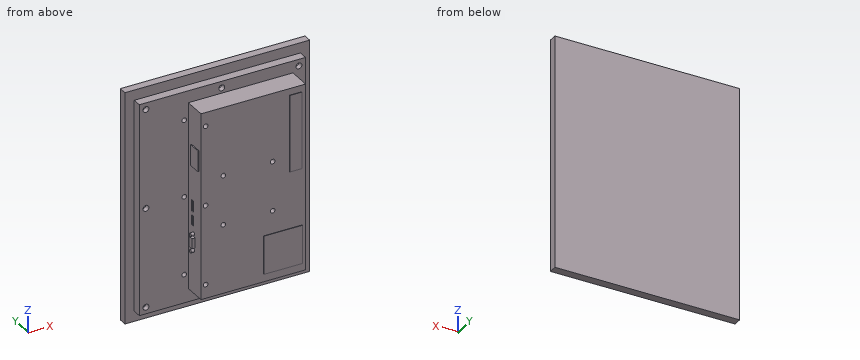
Autodesk Inventor part; units mm, degrees
ref_plane "YZ Plane" through (0, 0, 0) normal (1, 0, 0) x (0, 1, 0)
ref_plane "XZ Plane" through (0, 0, 0) normal (0, 1, 0) x (-1, 0, 0)
ref_plane "XY Plane" through (0, 0, 0) normal (0, 0, 1) x (1, 0, 0)
sketch "Sketch1" plane through (0, 0, 0) normal (0, 1, 0) x (-1, 0, 0)
  point P0 (0, 0)
sketch "Sketch2" plane through (0, 0, 0) normal (0, 1, 0) x (-1, 0, 0)
  line L0 (-139.5, 175.3) -> (139.5, 175.3)
  line L1 (139.5, 175.3) -> (139.5, -175.3)
  line L2 (139.5, -175.3) -> (-139.5, -175.3)
  line L3 (-139.5, -175.3) -> (-139.5, 175.3)
  line L4 (-139.5, 175.3) -> (139.5, -175.3) construction
  line L5 (139.5, 175.3) -> (-139.5, -175.3) construction
  point P0 (0, 0)
  dimension "d0" = 350.6
  dimension "d1" = 279
extrude "Extrusion1" add sketch "Sketch2" along normal blind 12.4
sketch "Sketch3" plane through (0, 0, 0) normal (0, -1, 0) x (1, 0, 0)
  line L0 (-125.5, -159.875) -> (125.5, -159.875)
  line L1 (125.5, -159.875) -> (125.5, 159.875)
  line L2 (125.5, 159.875) -> (-125.5, 159.875)
  line L3 (-125.5, 159.875) -> (-125.5, -159.875)
  line L4 (-125.5, -159.875) -> (125.5, 159.875) construction
  line L5 (125.5, -159.875) -> (-125.5, 159.875) construction
  point P0 (0, 0)
  dimension "d4" = 319.75
  dimension "d5" = 251
extrude "Extrusion2" add sketch "Sketch3" along normal blind 13.5
sketch "Sketch4" plane through (0, -13.5, 0) normal (0, -1, 0) x (1, 0, 0)
  line L0 (125.5, 159.875) -> (-125.5, 159.875)
  line L1 (-125.5, 159.875) -> (-125.5, -159.875)
  line L2 (125.5, -159.875) -> (125.5, 159.875)
  line L3 (-125.5, -159.875) -> (125.5, -159.875)
  point P0 (0, 0)
  point P1 (-115.5, 149.875)
  point P2 (-115.5, -149.875)
  point P3 (115.5, 149.875)
  point P4 (115.5, -149.875)
  dimension "d15" = 10
  dimension "d16" = 10
  dimension "d19" = 299.75
  dimension "d22" = 231
  dimension "d25" = 10
  dimension "d26" = 10
hole "Hole1" at (-115.5, -13.5, 149.875) at (115.5, -13.5, 149.875) at (115.5, -13.5, -149.875) at (-115.5, -13.5, -149.875) direction (0, 1, 0) diameter 9 depth 8 tip angle 118
sketch "Sketch5" plane through (0, -13.5, 0) normal (0, -1, 0) x (1, 0, 0)
  line L0 (125.5, 159.875) -> (-125.5, 159.875)
  line L1 (-125.5, 159.875) -> (-125.5, -159.875)
  line L2 (125.5, -159.875) -> (125.5, 159.875)
  point P0 (0, 0)
  point P1 (-115.5, 0)
  point P2 (115.5, 0)
  dimension "d34" = 159.875
  dimension "d35" = 10
  dimension "d38" = 231
  dimension "d43" = 10
hole "Hole2" at (-115.5, -13.5, 0) at (115.5, -13.5, 0) direction (0, 1, 0) diameter 9 depth 8 tip angle 118
sketch "Sketch6" plane through (0, -13.5, 0) normal (0, -1, 0) x (1, 0, 0)
  circle A0 centre (-115.5, 149.875) radius 4.5
  line L0 (-125.5, 159.875) -> (-125.5, -159.875)
  line L1 (-125.5, -159.875) -> (125.5, -159.875)
  line L2 (125.5, 159.875) -> (-125.5, 159.875)
  point P0 (0, 0)
  point P1 (-1, 149.875)
  point P2 (-1, -149.875)
  dimension "d55" = 298
  dimension "d52" = 124.5
  dimension "d60" = 10
  dimension "d188" = 10
hole "Hole3" at (-1, -13.5, -149.875) at (-1, -13.5, 149.875) direction (0, 1, 0) diameter 9 depth 8 tip angle 118
sketch "Sketch7" plane through (0, -13.5, 0) normal (0, -1, 0) x (1, 0, 0)
  line L0 (-51.5, 141.825) -> (106.5, 141.825)
  line L1 (106.5, 141.825) -> (106.5, -139.875)
  line L2 (106.5, -139.875) -> (-51.5, -139.875)
  line L3 (-51.5, -139.875) -> (-51.5, 141.825)
  line L4 (-51.5, 141.825) -> (106.5, -139.875) construction
  line L5 (106.5, 141.825) -> (-51.5, -139.875) construction
  line L6 (125.5, -159.875) -> (125.5, 159.875)
  line L7 (-125.5, -159.875) -> (125.5, -159.875)
  point P0 (0, 0)
  dimension "d61" = 281.7
  dimension "d62" = 158
  dimension "d63" = 19
  dimension "d64" = 20
extrude "Extrusion3" add sketch "Sketch7" along normal blind 33.6
sketch "Sketch8" plane through (0, -47.1, 0) normal (0, -1, 0) x (1, 0, 0)
  line L0 (100.2, 131.825) -> (82.2, 131.825)
  line L1 (82.2, 131.825) -> (82.2, 15.825)
  line L2 (82.2, 15.825) -> (100.2, 15.825)
  line L3 (100.2, 15.825) -> (100.2, 131.825)
  line L4 (100.2, 131.825) -> (82.2, 15.825) construction
  line L5 (82.2, 131.825) -> (100.2, 15.825) construction
  line L6 (106.5, -139.875) -> (106.5, 141.825)
  line L7 (106.5, 141.825) -> (-51.5, 141.825)
  point P0 (0, 0)
  point P1 (91.2, 73.825)
  dimension "d67" = 116
  dimension "d68" = 18
  dimension "d69" = 6.3
  dimension "d70" = 10
extrude "Extrusion4" add sketch "Sketch8" along normal blind 1
sketch "Sketch9" plane through (0, -47.1, 0) normal (0, -1, 0) x (1, 0, 0)
  line L0 (101, -70.275) -> (43.15, -70.275)
  line L1 (43.15, -70.275) -> (43.15, -128.125)
  line L2 (43.15, -128.125) -> (101, -128.125)
  line L3 (101, -128.125) -> (101, -70.275)
  line L4 (101, -70.275) -> (43.15, -128.125) construction
  line L5 (43.15, -70.275) -> (101, -128.125) construction
  line L6 (106.5, -139.875) -> (106.5, 141.825)
  line L7 (-51.5, -139.875) -> (106.5, -139.875)
  point P0 (0, 0)
  point P1 (72.075, -99.2)
  dimension "d73" = 5.5
  dimension "d74" = 57.85
  dimension "d75" = 11.75
  dimension "d76" = 57.85
extrude "Extrusion5" add sketch "Sketch9" along normal blind 1
sketch "Sketch10" plane through (0, -47.1, 0) normal (0, -1, 0) x (1, 0, 0)
  line L0 (106.5, 141.825) -> (-51.5, 141.825)
  line L1 (-51.5, 141.825) -> (-51.5, -139.875)
  line L2 (-51.5, -139.875) -> (106.5, -139.875)
  point P0 (0, 0)
  point P1 (-44.5, 121.025)
  point P2 (-44.5, -119.075)
  dimension "d86" = 20.8
  dimension "d87" = 7
  dimension "d90" = 240.1
  dimension "d95" = 20.8
hole "Hole4" at (-44.5, -47.1, 121.025) at (-44.5, -47.1, -119.075) direction (0, 1, 0) diameter 7 depth 8 tip angle 118
sketch "Sketch11" plane through (0, -47.1, 0) normal (0, -1, 0) x (1, 0, 0)
  line L0 (106.5, 141.825) -> (-51.5, 141.825)
  line L1 (-51.5, 141.825) -> (-51.5, -139.875)
  line L2 (125.5, 159.875) -> (-125.5, 159.875)
  point P0 (0, 0)
  point P1 (-44.5, 0.825)
  dimension "d103" = 141
  dimension "d104" = 7
  dimension "d185" = 159.05
hole "Hole5" at (-44.5, -47.1, 0.825) direction (0, 1, 0) diameter 7 depth 8 tip angle 118
sketch "Sketch12" plane through (0, -47.1, 0) normal (0, -1, 0) x (1, 0, 0)
  line L0 (106.5, 141.825) -> (-51.5, 141.825)
  line L1 (-51.5, 141.825) -> (-51.5, -139.875)
  point P0 (0, 0)
  point P1 (-17.7, 38.475)
  point P2 (-17.7, -36.025)
  point P3 (56.8, 38.475)
  point P4 (56.8, -36.025)
  dimension "d112" = 103.35
  dimension "d113" = 33.8
  dimension "d116" = 74.5
  dimension "d119" = 74.5
hole "Hole6" at (-17.7, -47.1, 38.475) at (56.8, -47.1, 38.475) at (56.8, -47.1, -36.025) at (-17.7, -47.1, -36.025) direction (0, 1, 0) diameter 7 depth 8 tip angle 118
sketch "Sketch13" plane through (-51.5, -13.5, -139.875) normal (-1, 0, 0) x (0, 0, 1)
  line L0 (223, -27.9) -> (191.35, -27.9)
  line L1 (191.35, -27.9) -> (191.35, -8.5)
  line L2 (191.35, -8.5) -> (223, -8.5)
  line L3 (223, -8.5) -> (223, -27.9)
  line L4 (223, -27.9) -> (191.35, -8.5) construction
  line L5 (191.35, -27.9) -> (223, -8.5) construction
  line L6 (281.7, 0) -> (281.7, -33.6)
  line L7 (281.7, -33.6) -> (0, -33.6)
  point P0 (139.875, 13.5)
  point P1 (207.175, -18.2)
  dimension "d122" = 58.7
  dimension "d123" = 31.65
  dimension "d124" = 19.4
  dimension "d133" = 5.7
extrude "Extrusion6" add sketch "Sketch13" along normal blind 1.5
sketch "Sketch14" plane through (-51.5, -13.5, -139.875) normal (-1, 0, 0) x (0, 0, 1)
  line L0 (139.25, -14.2) -> (122.25, -14.2)
  line L1 (122.25, -14.2) -> (122.25, -8)
  line L2 (122.25, -8) -> (139.25, -8)
  line L3 (139.25, -8) -> (139.25, -14.2)
  line L4 (139.25, -14.2) -> (122.25, -8) construction
  line L5 (122.25, -14.2) -> (139.25, -8) construction
  line L6 (191.35, -8.5) -> (191.35, -27.9)
  line L7 (281.7, -33.6) -> (0, -33.6)
  line L8 (191.35, -27.9) -> (223, -27.9)
  line L9 (299.75, 0) -> (-20, 0)
  line L10 (223, -8.5) -> (191.35, -8.5)
  point P0 (139.875, 13.5)
  point P1 (130.75, -11.1)
  dimension "d127" = 52.1
  dimension "d128" = 6.2
  dimension "d129" = 17
  dimension "d130" = 19.4
  dimension "d131" = 5.7
  dimension "d132" = 8.5
extrude "Extrusion7" cut sketch "Sketch14" against normal blind 1.5
sketch "Sketch15" plane through (-51.5, -13.5, -139.875) normal (-1, 0, 0) x (0, 0, 1)
  line L0 (116.35, -14.2) -> (101.55, -14.2)
  line L1 (101.55, -14.2) -> (101.55, -8)
  line L2 (101.55, -8) -> (116.35, -8)
  line L3 (116.35, -8) -> (116.35, -14.2)
  line L4 (116.35, -14.2) -> (101.55, -8) construction
  line L5 (101.55, -14.2) -> (116.35, -8) construction
  line L6 (122.25, -14.2) -> (122.25, -8)
  line L7 (281.7, -33.6) -> (0, -33.6)
  point P0 (139.875, 13.5)
  point P1 (108.95, -11.1)
  dimension "d136" = 5.9
  dimension "d137" = 6.2
  dimension "d138" = 14.8
  dimension "d141" = 19.4
extrude "Extrusion8" cut sketch "Sketch15" against normal blind 1.5
sketch "Sketch16" plane through (-51.5, -13.5, -139.875) normal (-1, 0, 0) x (0, 0, 1)
  circle A0 centre (90.05, -14.2) radius 2.5
  line L0 (101.55, -14.2) -> (101.55, -8)
  line L1 (281.7, -33.6) -> (0, -33.6)
  circle A1 centre (65.05, -14.2) radius 2.5
  point P0 (139.875, 13.5)
  dimension "d142" = 11.5
  dimension "d143" = 19.4
  dimension "d144" = 5
  dimension "d147" = 25
extrude "Extrusion9" add sketch "Sketch16" along normal blind 5
sketch "Sketch17" plane through (-51.5, -13.5, -139.875) normal (-1, 0, 0) x (0, 0, 1)
  line L0 (86.05, -18.35) -> (70.65, -18.35)
  line L1 (70.65, -18.35) -> (70.65, -10.05)
  line L2 (70.65, -10.05) -> (86.05, -10.05)
  line L3 (86.05, -10.05) -> (86.05, -18.35)
  line L4 (86.05, -18.35) -> (70.65, -10.05) construction
  line L5 (70.65, -18.35) -> (86.05, -10.05) construction
  line L6 (101.55, -14.2) -> (101.55, -8)
  line L7 (281.7, -33.6) -> (0, -33.6)
  point P0 (139.875, 13.5)
  point P1 (78.35, -14.2)
  dimension "d154" = 8.3
  dimension "d155" = 15.4
  dimension "d156" = 15.5
  dimension "d157" = 19.4
extrude "Extrusion10" add sketch "Sketch17" along normal blind 5
sketch "Sketch18" plane through (0, -13.5, 0) normal (0, -1, 0) x (1, 0, 0)
  line L0 (125.5, 159.875) -> (-125.5, 159.875)
  line L1 (-125.5, 159.875) -> (-125.5, -159.875)
  line L2 (-125.5, -159.875) -> (125.5, -159.875)
  point P0 (0, 0)
  point P1 (-57.6, 117.025)
  point P2 (-57.6, -117.025)
  dimension "d167" = 42.85
  dimension "d168" = 67.9
  dimension "d171" = 234.05
  dimension "d176" = 42.85
hole "Hole7" at (-57.6, -13.5, 117.025) at (-57.6, -13.5, -117.025) direction (0, 1, 0) diameter 7 depth 8 tip angle 118
sketch "Sketch19" plane through (0, -13.5, 0) normal (0, -1, 0) x (1, 0, 0)
  circle A0 centre (-57.6, 117.025) radius 3.5
  line L0 (125.5, 159.875) -> (-125.5, 159.875)
  line L1 (-125.5, 159.875) -> (-125.5, -159.875)
  point P0 (0, 0)
  point P1 (-57.6, 0.825)
  dimension "d186" = 159.05
  dimension "d187" = 67.9
hole "Hole8" at (-57.6, -13.5, 0.825) direction (0, 1, 0) diameter 7 depth 8 tip angle 118
properties part number "LCDScreen"
The listing builds one solid part. Answer for the finished solid, in the listing's coordinates (mm). Coordinates: 2 decimals unless noted, no trailing zeros. Order: outer loops, then holes, each group sorted by start corner. A loop starts at its lowest first (then second) coordinate and runs counter-clockwise, first axis right, second up.
Q1. A cutting plane is placed at C-C, the plane x = -83. Write down the section's boundary in (y, z) (3 decimals), and give its area (3 significant figures).
Q2. A cutting plane is placed at B-B, the plane z = 70.5. Write down the section's boundary in (x, y), and give its area (3 significant figures).
Q3. Given P1, Ø5, axis at x = 22.5, y = -37, coming from the -Z side (3 decimals); P2, Ø8, axis at y = -34.5, z = 59.5, coming from the -X side; P3, Ø5.5, axis at x = -44.5, z = -119.075, coming from the -Y side; P4, Ø15, axis at y = -4.5, z = 58, coming from the -X side, each flat-ended and moving along its own axis, determine where each tip first touches the part or whether it passes through.
Q4. Consider line 1 (Z direction, x = 115, y = -9) (3 decimals); line 2 (Z direction, x = -115.5, y = -10) (3 decimals); line 3 (Z direction, x = -1, y = -7) (3 decimals). Determine where each line is inside the solid, lowest interval first.
Q5. A cutting plane is placed at D-D, the plane z = 29. Write down the section's boundary in (x, y), and give its area (3 significant figures).
Q6. A cutting plane is placed at A-A, the plane x = 23. Write down the section's boundary in (y, z) (3 decimals), and give its area (3 significant figures).
Answers follow:
1. outline: (-13.5, -159.875) - (0, -159.875) - (0, -175.3) - (12.4, -175.3) - (12.4, 175.3) - (0, 175.3) - (0, 159.875) - (-13.5, 159.875) - close
1. area: 8,660 mm2
2. outline: (-139.5, 0) - (-125.5, 0) - (-125.5, -13.5) - (-51.5, -13.5) - (-51.5, -22) - (-53, -22) - (-53, -41.4) - (-51.5, -41.4) - (-51.5, -47.1) - (82.2, -47.1) - (82.2, -48.1) - (100.2, -48.1) - (100.2, -47.1) - (106.5, -47.1) - (106.5, -13.5) - (125.5, -13.5) - (125.5, 0) - (139.5, 0) - (139.5, 12.4) - (-139.5, 12.4) - close
2. area: 12,200 mm2
3. P1: stops at z = -139.875
3. P2: stops at x = -53
3. P3: stops at y = -38.65
3. P4: stops at x = -139.5
4. line 1: z = -159.875 to -154.347, -145.403 to -4.472, 4.472 to 145.403, 154.347 to 159.875
4. line 2: z = -159.875 to -154.375, -145.375 to -4.5, 4.5 to 145.375, 154.375 to 159.875
4. line 3: z = -159.875 to -154.375, -145.375 to 145.375, 154.375 to 159.875
5. outline: (-139.5, 0) - (-125.5, 0) - (-125.5, -13.5) - (-51.5, -13.5) - (-51.5, -47.1) - (82.2, -47.1) - (82.2, -48.1) - (100.2, -48.1) - (100.2, -47.1) - (106.5, -47.1) - (106.5, -13.5) - (125.5, -13.5) - (125.5, 0) - (139.5, 0) - (139.5, 12.4) - (-139.5, 12.4) - close
5. area: 12,200 mm2
6. outline: (-47.1, -139.875) - (-13.5, -139.875) - (-13.5, -159.875) - (0, -159.875) - (0, -175.3) - (12.4, -175.3) - (12.4, 175.3) - (0, 175.3) - (0, 159.875) - (-13.5, 159.875) - (-13.5, 141.825) - (-47.1, 141.825) - close
6. area: 18,100 mm2
